The listing builds one solid part. Answer for the finished solid, in the listing's coordinates (mm). A direction names the side the tool comes from. Round coordinates to 2 decimals unless told otherwise and drop trailing zeros. Write each loop counter-clockwise with the first axis right and the second up, starting at its lowest first coordinate (ties: lowest second). Pieces come first, ordered by that corner, then holes. Notation, with made-up numbers: (8.25, -15.5) - (38.25, -15.5) arc R16 cw to (38.25, -4.5) - close; hole circle Ø6 at (29.25, 84). An arc over 180 degrees is marked (long way). Return JSON: item names as keys, results as strings. Group by question number.
(1) Section B-B, the plane z = 2.75 is taken. Write down the section's boundary in (x, y).
(2) Which of the six approach directions +Z, -Z, +X, -X, +Y, -Y give full straight-line access (tool end or side, diameter ignored) to faces 5 (the flat face through (11, -2, -2)), 6 (the flat face through (17.05, -2, 0)), 7 (the flat face through (2, -2, 2))?
(3) Section C-C, the plane x = 14.65 is taken. Write down the section's boundary in (y, z).
(4) Each of these flat-tipped pins is pushed along its axis until it touches: pin 1 (3 mm diameter, centred on y = -2, z = -0.5, fed in from +X); pin 2 (3 mm diameter, centred on x = 13, z = -0.5, fed in from -Y); pin 3 (2 mm diameter, centred on x = 7.5, z = -1.5, fed in from +Y). Where does it stop, or does it pass through?
(5) Section A-A, the plane y = 2.35 is taken. Write down the section's boundary in (x, z), then the cut area to 3 significant figures.
(6) Determine the mould class of faces 1 (the flat face through (11, 12, 1.55)), 2 (the flat face through (2.35, -2, 0)), 3 (the cylindrical face through (15.747, 2.695, -0.045)), 4 (the cylindrical face through (0.301, 9.365, 0.045)) for opening direction X: +X half, -X half, draft (parallel to the pull), parting line (faces both ways), or undercut.
(7) Find the intervals of material crossed by line 1 along Y through (x, z) = (5, 2.25); line 2 along Y through (x, z) = (14.65, 0.5); line 3 along Y through (x, z) = (2.5, -2.25), in increasing order. Write a range as [from, to].
(8) Section D-D, the plane z = -0.75 is taken. Give the number of separate pieces and of enclosed holes in the cut face, then the cut area to 3 significant figures.
```python
from build123d import *

# Parameters (mm, degrees)
F0_R     = 1.15
F1_DEPTH = 3.2
F3_DEPTH = 1.55
F4_W     = 0.8
F4_H     = 3.6
F5_DEPTH = 2
F7_DEPTH = 1.55


with BuildPart() as f1:
    # F0 (on Top) → F1 (new body, symmetric)
    with BuildSketch(Plane.XY):
        with BuildLine():
            ThreePointArc((0, 1), (0.292893, 0.292893), (1, 0))
            Line((1, 0), (18.9, 0))
            ThreePointArc((18.9, 0), (19.607107, 0.292893), (19.9, 1))
            Line((19.9, 1), (19.9, 8.65))
            ThreePointArc((19.9, 8.65), (19.607107, 9.357107), (18.9, 9.65))
            Line((18.9, 9.65), (1, 9.65))
            ThreePointArc((1, 9.65), (0.292893, 9.357107), (0, 8.65))
            Line((0, 8.65), (0, 1))
        make_face()
        with BuildLine():
            ThreePointArc((5.05, 1.2), (3.9, 2.35), (5.05, 3.5))
            Line((5.05, 3.5), (5.25, 3.5))
            ThreePointArc((5.25, 3.5), (6.4, 2.35), (5.25, 1.2))
            Line((5.25, 1.2), (5.05, 1.2))
        make_face(mode=Mode.SUBTRACT)
        with Locations((14.65, 2.35)):
            Circle(F0_R, mode=Mode.SUBTRACT)
    extrude(amount=F1_DEPTH, both=True)

    # F2 (on Top) → F3 (join, symmetric)
    with BuildSketch(Plane.XY):
        with BuildLine():
            Line((5.95, 9.65), (8.35, 9.65))
            ThreePointArc((8.35, 9.65), (7.15, 10.45), (5.95, 9.65))
        make_face()
    extrude(amount=F3_DEPTH, both=True)

    # F4 (on Top) → F5 (join, symmetric)
    with BuildSketch(Plane.XY):
        with Locations((17.45, -1.8)):
            Rectangle(F4_W, F4_H)
        with Locations((10.8, -1.8)):
            Rectangle(F4_W, F4_H)
        with Locations((1.95, -1.8)):
            Rectangle(F4_W, F4_H)
    extrude(amount=F5_DEPTH, both=True)

    # F6 (on Top) → F7 (join, symmetric)
    with BuildSketch(Plane.XY):
        Polygon((19.028934, 14.071202), (18.884875, 14.55), (1.64816, 9.363898), (1.792219, 8.8851), align=None)
    extrude(amount=F7_DEPTH, both=True)


solid = f1.part
```
Working result:
{
 "1": {"outline": "(0, 1) arc R1 ccw to (1, 0) - (18.9, 0) arc R1 ccw to (19.9, 1) - (19.9, 8.65) arc R1 ccw to (18.9, 9.65) - (1, 9.65) arc R1 ccw to (0, 8.65) - close; hole (5.05, 1.2) - (5.25, 1.2) arc R1.15 ccw to (5.25, 3.5) - (5.05, 3.5) arc R1.15 ccw to start; hole circle Ø2.3 at (14.65, 2.35)"},
 "2": {"face 5": "-Z, +X, -X, -Y", "face 6": "+Z, -Z, -Y", "face 7": "+Z, +X, -X, -Y"},
 "3": {"outline": "(0, -3.2) - (1.2, -3.2) - (1.2, 3.2) - (0, 3.2) - close; (3.5, -3.2) - (9.65, -3.2) - (9.65, 3.2) - (3.5, 3.2) - close; (12.75, -1.55) - (13.28, -1.55) - (13.28, 1.55) - (12.75, 1.55) - close"},
 "4": {"pin 1": "stops at x = 17.85", "pin 2": "stops at y = 0", "pin 3": "stops at y = 11.43"},
 "5": {"outline": "(0, -3.2) - (3.9, -3.2) - (3.9, 3.2) - (0, 3.2) - close; (6.4, -3.2) - (13.5, -3.2) - (13.5, 3.2) - (6.4, 3.2) - close; (15.8, -3.2) - (19.9, -3.2) - (19.9, 3.2) - (15.8, 3.2) - close", "area": "96.6 mm^2"},
 "6": {"face 1": "draft", "face 2": "undercut", "face 3": "undercut", "face 4": "-X half"},
 "7": {"line 1": "y = [0, 1.2], [3.5, 9.65]", "line 2": "y = [0, 1.2], [3.5, 9.65], [12.75, 13.28]", "line 3": "y = [0, 9.65]"},
 "8": {"separate pieces": "1", "enclosed holes": "3", "area": "201 mm^2"}
}
